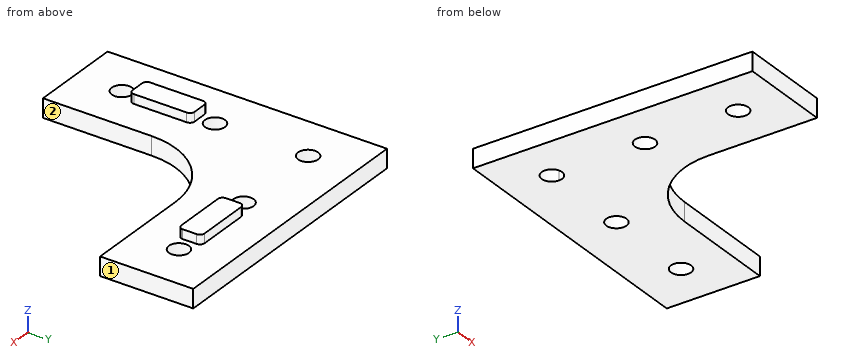
from build123d import *

# Parameters (mm, degrees)
F1_DEPTH = 6
F2_R     = 3.25
F3_DEPTH = 8
F5_DEPTH = 3


with BuildPart() as f1:
    # F0 (on Top) → F1 (new body)
    with BuildSketch(Plane.XY):
        with BuildLine():
            Line((-28.6977304518, 102.8932180628), (-58.6977304518, 102.8932180628))
            Line((-58.6977304518, 102.8932180628), (-58.6977304518, 72.8932180628))
            Line((-58.6977304518, 72.8932180628), (-58.6977304518, 12.8932180628))
            Line((-58.6977304518, 12.8932180628), (-28.6977304518, 12.8932180628))
            Line((-28.6977304518, 12.8932180628), (-28.6977304518, 47.8932180628))
            ThreePointArc((-28.6977304518, 47.8932180628), (-21.3753999815, 65.5708875925), (-3.6977304518, 72.8932180628))
            Line((-3.6977304518, 72.8932180628), (31.3022695482, 72.8932180628))
            Line((31.3022695482, 72.8932180628), (31.3022695482, 102.8932180628))
            Line((31.3022695482, 102.8932180628), (-28.6977304518, 102.8932180628))
        make_face()
    extrude(amount=F1_DEPTH)

    # F2 (on face) → F3 (cut)
    with BuildSketch(Plane.XY.offset(6)):
        with Locations((-13.6977304518, 87.8932180628)):
            Circle(F2_R)
        with Locations((16.3022695482, 87.8932180628)):
            Circle(F2_R)
        with Locations((-43.6977304518, 57.8932180628)):
            Circle(F2_R)
        with Locations((-43.6977304518, 27.8932180628)):
            Circle(F2_R)
        with BuildLine():
            Line((-45.9958274907, 90.1913151017), (-41.399633413, 85.595121024))
            ThreePointArc((-41.399633413, 85.595121024), (-40.6951219712, 86.6494969076), (-40.4477304518, 87.8932180628))
            ThreePointArc((-40.4477304518, 87.8932180628), (-42.4540092966, 90.8958265435), (-45.9958274907, 90.1913151017))
        make_face()
        with BuildLine():
            ThreePointArc((-45.9958274907, 90.1913151017), (-45.9958274907, 85.595121024), (-41.399633413, 85.595121024))
            Line((-41.399633413, 85.595121024), (-45.9958274907, 90.1913151017))
        make_face()
    extrude(amount=-F3_DEPTH, mode=Mode.SUBTRACT)

    # F4 (on face) → F5 (join)
    with BuildSketch(Plane.XY.offset(6)):
        with BuildLine():
            Line((9.8022695482, 91.6432180628), (-7.1977304518, 91.6432180628))
            ThreePointArc((-7.1977304518, 91.6432180628), (-8.2583906236, 91.2038782346), (-8.6977304518, 90.1432180628))
            Line((-8.6977304518, 90.1432180628), (-8.6977304518, 85.6432180628))
            ThreePointArc((-8.6977304518, 85.6432180628), (-8.2583906236, 84.582557891), (-7.1977304518, 84.1432180628))
            Line((-7.1977304518, 84.1432180628), (9.8022695482, 84.1432180628))
            ThreePointArc((9.8022695482, 84.1432180628), (10.86292972, 84.582557891), (11.3022695482, 85.6432180628))
            Line((11.3022695482, 85.6432180628), (11.3022695482, 90.1432180628))
            ThreePointArc((11.3022695482, 90.1432180628), (10.86292972, 91.2038782346), (9.8022695482, 91.6432180628))
        make_face()
        with BuildLine():
            Line((-41.4477304518, 52.8932180628), (-45.9477304518, 52.8932180628))
            ThreePointArc((-45.9477304518, 52.8932180628), (-47.0083906236, 52.4538782346), (-47.4477304518, 51.3932180628))
            Line((-47.4477304518, 51.3932180628), (-47.4477304518, 34.3932180628))
            ThreePointArc((-47.4477304518, 34.3932180628), (-47.0083906236, 33.332557891), (-45.9477304518, 32.8932180628))
            Line((-45.9477304518, 32.8932180628), (-41.4477304518, 32.8932180628))
            ThreePointArc((-41.4477304518, 32.8932180628), (-40.38707028, 33.332557891), (-39.9477304518, 34.3932180628))
            Line((-39.9477304518, 34.3932180628), (-39.9477304518, 51.3932180628))
            ThreePointArc((-39.9477304518, 51.3932180628), (-40.38707028, 52.4538782346), (-41.4477304518, 52.8932180628))
        make_face()
    extrude(amount=F5_DEPTH)


solid = f1.part
Source: CAD feature listing. Evaluate the final solid. Frame: model axes, mm. Face numbers are marked on the shaded views. A direction names the side the tool comes from. Give positions to 0.01 mm unless a question says otherwise; leave off trailing zeros. Write each loop counter-clockwise with the first axis right and the second up, starting at its lowest first coordinate (ties: lowest second). Pieces come first, ordered by that corner, then holes. Notation, with made-up numbers: (54.5, 52.25) - (64.5, 52.25) arc R32 cw to (64.5, 83.25) - close; hole circle Ø2 at (-31.5, 28). An arc over 180 degrees is marked (long way). Write item = value, one per line. Start each with the question number.
Q1. Cut plane C-C, the plane x = 8. Return loops of the section in (y, z), then the cut area to 4 significant figures.
Q2. Material intervals for probe 1 along Y at (x, z) = (-46, 2.75); probe 2 along Z at (x, y) = (-36, 76); probe 3 along X at (y, z) = (45.5, 3), sorted ascending.
Q3. Reachability of the marked faces 1 and 2 from +Z, -Z, +X, -X, +Y, -Y: full face, straight path, thin tool, end or side. Return the list, or none.
Q4. Cut plane A-A, the plane z = 7.5. Return loops of the section in (x, y), then the cut area to 3 significant figures.
Q5. Cut plane D-D, the plane z = 3. Return loops of the section in (x, y).
Q6. Cut plane B-B, the plane y = 30. Return loops of the section in (x, z), then the cut area to 3 significant figures.
Q7. Pin query (flat end, axial travel): pin 1 Ø1.8 at (x, z) = (11, 2) entering from -Y; pin 2 Ø3 at (x, y) = (-31, 47.5) entering from +Z; pin 3 Ø5 at (x, y) = (-43.7, 27.89) entering from +Z; pin 4 Ø0.9 at (y, z) = (40, 7) entering from -X. Return the tip coordinate at first contact, or that it passes through.
Computed values:
q1.outline = (72.89, 0) - (102.89, 0) - (102.89, 6) - (91.64, 6) - (91.64, 9) - (84.14, 9) - (84.14, 6) - (72.89, 6) - close
q1.area = 202.5 mm²
q2.probe_1 = 12.89 to 25.6, 30.19 to 55.6, 60.19 to 85.6, 90.19 to 102.89
q2.probe_2 = 0 to 6
q2.probe_3 = -58.7 to -28.7
q3.face_1 = +Z, -Z, +X, +Y, -Y
q3.face_2 = +Z, -Z, +X, -Y
q4.outline = (-47.45, 34.39) arc R1.5 ccw to (-45.95, 32.89) - (-41.45, 32.89) arc R1.5 ccw to (-39.95, 34.39) - (-39.95, 51.39) arc R1.5 ccw to (-41.45, 52.89) - (-45.95, 52.89) arc R1.5 ccw to (-47.45, 51.39) - close; (-8.7, 85.64) arc R1.5 ccw to (-7.2, 84.14) - (9.8, 84.14) arc R1.5 ccw to (11.3, 85.64) - (11.3, 90.14) arc R1.5 ccw to (9.8, 91.64) - (-7.2, 91.64) arc R1.5 ccw to (-8.7, 90.14) - close
q4.area = 296 mm²
q5.outline = (-58.7, 12.89) - (-28.7, 12.89) - (-28.7, 47.89) arc R25 cw to (-3.7, 72.89) - (31.3, 72.89) - (31.3, 102.89) - (-58.7, 102.89) - close; hole circle Ø6.5 at (-43.7, 27.89); hole circle Ø6.5 at (-43.7, 57.89); hole circle Ø6.5 at (-43.7, 87.89); hole circle Ø6.5 at (-13.7, 87.89); hole circle Ø6.5 at (16.3, 87.89)
q6.outline = (-58.7, 0) - (-46.17, 0) - (-46.17, 6) - (-58.7, 6) - close; (-41.22, 0) - (-28.7, 0) - (-28.7, 6) - (-41.22, 6) - close
q6.area = 150 mm²
q7.pin_1 = 72.89
q7.pin_2 = 6
q7.pin_3 = through
q7.pin_4 = -47.45
